```python
from build123d import *

# Parameters (mm, degrees)
SKETCH1_W           = 30
SKETCH1_H           = 30
BOSS_EXTRUDE1_DEPTH = 3
SKETCH2_R           = 15
BOSS_EXTRUDE2_DEPTH = 7
BOSS_EXTRUDE3_DEPTH = 7
FILLET1_R           = 3
SKETCH5_R           = 14.15
CUT_EXTRUDE2_DEPTH  = 10
SKETCH6_R           = 1.5
CUT_EXTRUDE3_DEPTH  = 10
SKETCH7_R           = 8
BOSS_EXTRUDE4_DEPTH = 1.5
SKETCH8_W           = 13.15764426
SKETCH8_H           = 1.5
BOSS_EXTRUDE5_DEPTH = 1.5
SKETCH9_R           = 0.75
CUT_EXTRUDE4_DEPTH  = 1.5
SKETCH10_R          = 2
CUT_EXTRUDE5_DEPTH  = 1
SKETCH11_R          = 6.75
CUT_EXTRUDE6_DEPTH  = 0.5
SKETCH12_W          = 3.4
SKETCH12_H          = 2.5
CUT_EXTRUDE7_DEPTH  = 0.5
CUT_EXTRUDE8_DEPTH  = 0.5
SKETCH14_R          = 1
CUT_EXTRUDE9_DEPTH  = 2
FILLET2_R           = 0.5


with BuildPart() as part:
    # Sketch1 → Boss-Extrude1 (new body)
    with BuildSketch(Plane.XY):
        Rectangle(SKETCH1_W, SKETCH1_H)
    extrude(amount=BOSS_EXTRUDE1_DEPTH)

    # Sketch2 → Boss-Extrude2 (add)
    with BuildSketch(Plane.XY.offset(3)):
        Circle(SKETCH2_R)
    extrude(amount=BOSS_EXTRUDE2_DEPTH)

    # Sketch4 → Boss-Extrude3 (add)
    with BuildSketch(Plane.XY.offset(3)):
        with BuildLine():
            Line((-14.121320344, 9.878679656), (-4.242640687, 0))
            Line((-4.242640687, 0), (-14.121320344, -9.878679656))
            ThreePointArc((-14.121320344, -9.878679656), (-14.121320344, -14.121320344), (-9.878679656, -14.121320344))
            Line((-9.878679656, -14.121320344), (0, -4.242640687))
            Line((0, -4.242640687), (9.878679656, -14.121320344))
            ThreePointArc((9.878679656, -14.121320344), (14.121320344, -14.121320344), (14.121320344, -9.878679656))
            Line((14.121320344, -9.878679656), (4.242640687, 0))
            Line((4.242640687, 0), (14.121320344, 9.878679656))
            ThreePointArc((14.121320344, 9.878679656), (14.121320344, 14.121320344), (9.878679656, 14.121320344))
            Line((9.878679656, 14.121320344), (0, 4.242640687))
            Line((0, 4.242640687), (-9.878679656, 14.121320344))
            ThreePointArc((-9.878679656, 14.121320344), (-14.121320344, 14.121320344), (-14.121320344, 9.878679656))
        make_face()
    extrude(amount=BOSS_EXTRUDE3_DEPTH)

    # Fillet1
    fillet1_edges = [part.edges().sort_by_distance(p)[0] for p in [
        (-15, -15, 1.5),
        (15, -15, 1.5),
        (15, 15, 1.5),
        (-15, 15, 1.5),
    ]]
    fillet(fillet1_edges, radius=FILLET1_R - 0.0001)  # a hair under: the kernel refuses the full size

    # Sketch5 → Cut-Extrude2 (cut)
    with BuildSketch(Plane.XY.offset(10)):
        Circle(SKETCH5_R)
    extrude(amount=-CUT_EXTRUDE2_DEPTH, mode=Mode.SUBTRACT)

    # Sketch6 → Cut-Extrude3 (cut)
    with BuildSketch(Plane.XY.offset(10)):
        with Locations((-12, 12)):
            Circle(SKETCH6_R)
        with Locations((12, 12)):
            Circle(SKETCH6_R)
        with Locations((12, -12)):
            Circle(SKETCH6_R)
        with Locations((-12, -12)):
            Circle(SKETCH6_R)
    extrude(amount=-CUT_EXTRUDE3_DEPTH, mode=Mode.SUBTRACT)



with BuildPart() as body_2:
    # Sketch7 → Boss-Extrude4 (new body)
    with BuildSketch(Plane(origin=(0, 0, 0), x_dir=(-1, 0, 0), z_dir=(0, 0, -1))):
        Circle(SKETCH7_R)
    extrude(amount=-BOSS_EXTRUDE4_DEPTH)


with BuildPart() as part_1:
    add(part.part)

    add(body_2.part)  # Boss-Extrude5 merges body 2
    # Sketch8 → Boss-Extrude5 (add)
    with BuildSketch(Plane(origin=(0, 0, 0), x_dir=(-1, 0, 0), z_dir=(0, 0, -1))):
        Polygon((-0.061069882, -1.605776139), (-6.639892012, -13.000630322), (-7.938930118, -12.250630322), (-1.360107988, -0.855776139), align=None)
        with Locations((8, 0)):
            Rectangle(SKETCH8_W, SKETCH8_H)
        Polygon((-1.360107988, 0.855776139), (-7.938930118, 12.250630322), (-6.639892012, 13.000630322), (-0.061069882, 1.605776139), align=None)
    extrude(amount=-BOSS_EXTRUDE5_DEPTH)

    # Sketch9 → Cut-Extrude4 (cut)
    with BuildSketch(Plane(origin=(0, 0, 0), x_dir=(-1, 0, 0), z_dir=(0, 0, -1))):
        Circle(SKETCH9_R)
    extrude(amount=-CUT_EXTRUDE4_DEPTH, mode=Mode.SUBTRACT)

    # Sketch10 → Cut-Extrude5 (cut)
    with BuildSketch(Plane(origin=(0, 0, 0), x_dir=(-1, 0, 0), z_dir=(0, 0, -1))):
        Circle(SKETCH10_R)
    extrude(amount=-CUT_EXTRUDE5_DEPTH, mode=Mode.SUBTRACT)

    # Sketch11 → Cut-Extrude6 (cut)
    with BuildSketch(Plane(origin=(0, 0, 0), x_dir=(-1, 0, 0), z_dir=(0, 0, -1))):
        Circle(SKETCH11_R)
    extrude(amount=-CUT_EXTRUDE6_DEPTH, mode=Mode.SUBTRACT)

    # Sketch12 → Cut-Extrude7 (cut)
    with BuildSketch(Plane(origin=(0, 0, 0), x_dir=(-1, 0, 0), z_dir=(0, 0, -1))):
        with Locations((-8.1, -14.251318629)):
            Rectangle(SKETCH12_W, SKETCH12_H)
    extrude(amount=-CUT_EXTRUDE7_DEPTH, mode=Mode.SUBTRACT)

    # Sketch13 → Cut-Extrude8 (cut)
    with BuildSketch(Plane(origin=(0, 0, 0), x_dir=(-1, 0, 0), z_dir=(0, 0, -1))):
        Polygon((-1.799060557, -4.71606429), (-6.993041412, -13.712303025), (-7.685861735, -13.312303025), (-2.49188088, -4.31606429), align=None)
    extrude(amount=-CUT_EXTRUDE8_DEPTH, mode=Mode.SUBTRACT)

    # Sketch14 → Cut-Extrude9 (cut)
    with BuildSketch(Plane(origin=(0, 0, 0.5), x_dir=(-1, 0, 0), z_dir=(0, 0, -1))):
        with Locations((-2.291903498, -4.48287736)):
            Circle(SKETCH14_R)
    extrude(amount=-CUT_EXTRUDE9_DEPTH, mode=Mode.SUBTRACT)

    # Fillet2
    fillet2_edges = [part_1.edges().sort_by_distance(p)[0] for p in [
        (13.317472766, 9.074832079, 10),
        (14.121320344, 14.121320344, 10),
        (9.074832079, 13.317472766, 10),
        (-9.074832079, 13.317472766, 10),
        (-14.121320344, 14.121320344, 10),
        (-13.317472766, 9.074832079, 10),
        (-13.317472766, -9.074832079, 10),
        (-14.121320344, -14.121320344, 10),
        (-9.074832079, -13.317472766, 10),
        (9.074832079, -13.317472766, 10),
        (14.121320344, -14.121320344, 10),
        (13.317472766, -9.074832079, 10),
    ]]
    fillet(fillet2_edges, radius=FILLET2_R)


solid = part_1.part
```
Design review of the part built by this model. Coordinates are the model's own, in mm. A direction names the side the tool comes from. Coordinates: 2 decimals unless noted, no trailing zeros. Order: outer loops, then holes, each group sorted by start corner. A loop starts at its lowest first (then second) coordinate and runs counter-clockwise, first axis right, second up. Notation, with made-up numbers: (27.5, -35) -> (70.5, -35) arc R7 cw to (70.5, -23) -> close; hole circle Ø5 at (8.5, 70.5). An arc over 180 degrees is marked (long way). One line per item, written item: value. Start each with the question number.
Q1. Insertion check: pin 1 Ø3 at (x, y) = (1.5, 1) entering from -Z; pin 2 Ø3 at (x, y) = (2.29, -4.48) entering from +Z. Each pin has a flat end and moves straight along its axis. Give the tip position at first contact, or say it passes through.
Q2. Take a section at C-C, the plane x = -2.5. State the section outline as (y, z) points.
Q3. Take a section at B-B, the plane y = 1.5. State the section outline as (x, z) points, then the cut area to 3 significant figures.
Q4. Tool access review of faces 1 (the cylindrical face through (-15, 0, 6)), 2 (the flat face through (13.33, -9.09, 6.2)), 3 (the flat face through (-9.064, 13.306, 6.204)): name each direction out of +Z, -Z, +X, -X, +Y, -Y from which nothing blocks a thin tool from reaching the whole face with its end or side.
Q5. Mouldability with a two-part tool opening along Z and no side actions: class faces 4 (the cylindrical face through (-13.5, -11.93, 5.07)), 5 (the cylindrical face through (9.17, 13.2, 9.86)) as pulls with the +Z half, pulls with the -Z half, needs draft (parallel to the pull), parting line crosses it, or undercut.
Q6. For probe 1 along Y at (x, z) = (0, 0.8); probe 2 along Y at (x, z) = (0, 0.2); probe 3 along X at (y, z) = (13, 2.5), list the stretches that pass through material, from the lowest coordinate up.
Q7. Take a section at A-A, the plane z = 4.25. State the section outline as (x, y) points, then the cut area to 3 significant figures.
Values follow:
1. pin 1: stops at z = 0.5
1. pin 2: stops at z = 1.5
2. outline: (-15, 0) -> (-13.93, 0) -> (-13.93, 10) -> (-14.79, 10) -> (-14.79, 3) -> (-15, 3) -> close; (-7.6, 0) -> (-6.27, 0) -> (-6.27, 0.5) -> (6.27, 0.5) -> (6.27, 0) -> (7.6, 0) -> (7.6, 1.5) -> (-7.6, 1.5) -> close; (13.93, 0) -> (15, 0) -> (15, 3) -> (14.79, 3) -> (14.79, 10) -> (13.93, 10) -> close
3. outline: (-15, 0) -> (-14.07, 0) -> (-14.07, 10) -> (-14.92, 10) -> (-14.92, 3) -> (-15, 3) -> close; (-7.86, 0) -> (-6.58, 0) -> (-6.58, 0.5) -> (-1.32, 0.5) -> (-1.32, 1) -> (1.32, 1) -> (1.32, 0.5) -> (6.58, 0.5) -> (6.58, 0) -> (7.86, 0) -> (7.86, 1.5) -> (-7.86, 1.5) -> close; (14.07, 0) -> (15, 0) -> (15, 3) -> (14.92, 3) -> (14.92, 10) -> (14.07, 10) -> close
3. area: 33.2 mm2
4. face 1: +Z, -X
4. face 2: +Z, +X
4. face 3: +Z, +Y
5. face 4: needs draft
5. face 5: pulls with the +Z half
6. probe 1: y = -15 to -14.15, -8 to -2, 2 to 8, 14.15 to 15
6. probe 2: y = -15 to -14.15, -8 to -6.75, 6.75 to 8, 14.15 to 15
6. probe 3: x = -14.83 to -13.12, -10.88 to -5.59, 5.59 to 10.88, 13.12 to 14.83
7. outline: (-14.12, -9.88) arc R3 ccw to (-9.88, -14.12) -> (-8.27, -12.51) arc R15 ccw to (8.27, -12.51) -> (9.88, -14.12) arc R3 ccw to (14.12, -9.88) -> (12.51, -8.27) arc R15 ccw to (12.51, 8.27) -> (14.12, 9.88) arc R3 ccw to (9.88, 14.12) -> (8.27, 12.51) arc R15 ccw to (-8.27, 12.51) -> (-9.88, 14.12) arc R3 ccw to (-14.12, 9.88) -> (-12.51, 8.27) arc R15 ccw to (-12.51, -8.27) -> close; hole circle Ø28.3 at (0, 0); hole circle Ø3 at (-12, -12); hole circle Ø3 at (-12, 12); hole circle Ø3 at (12, -12); hole circle Ø3 at (12, 12)
7. area: 156 mm2
